The model under review builds one solid part; all positions refer to its coordinate system, in mm. A direction names the side the tool comes from. Round coordinates to 2 decimals unless told otherwise and drop trailing zeros. Order: outer loops, then holes, each group sorted by start corner. A loop starts at its lowest first (then second) coordinate and runs counter-clockwise, first axis right, second up.
```python
from build123d import *

# Parameters (mm, degrees)
SKETCH1_W                                           = 80
SKETCH1_H                                           = 100
BOSS_EXTRUDE1_DEPTH                                 = 10
SKETCH2_R                                           = 18
CUT_EXTRUDE1_DEPTH                                  = 129.452325787
SKETCH3_W                                           = 80
SKETCH3_H                                           = 46
CUT_EXTRUDE2_DEPTH                                  = 4
CBORE_FOR_M3_HEX_SOCKET_HEAD_CAP_SCREW1_D           = 3.4
CBORE_FOR_M3_HEX_SOCKET_HEAD_CAP_SCREW1_CBORE_D     = 6.5
CBORE_FOR_M3_HEX_SOCKET_HEAD_CAP_SCREW1_CBORE_DEPTH = 3.4


with BuildPart() as part:
    # Sketch1 → Boss-Extrude1 (new body)
    with BuildSketch(Plane.XY):
        with Locations((40, 50)):
            Rectangle(SKETCH1_W, SKETCH1_H)
    extrude(amount=BOSS_EXTRUDE1_DEPTH)

    # Sketch2 → Cut-Extrude1 (cut, through all)
    with BuildSketch(Plane.XY.offset(10)):
        with Locations((40, 73)):
            Circle(SKETCH2_R)
    extrude(amount=-CUT_EXTRUDE1_DEPTH, mode=Mode.SUBTRACT)

    # Sketch3 → Cut-Extrude2 (cut)
    with BuildSketch(Plane.XY.offset(10)):
        with Locations((40, 23)):
            Rectangle(SKETCH3_W, SKETCH3_H)
    extrude(amount=-CUT_EXTRUDE2_DEPTH, mode=Mode.SUBTRACT)

    # CBORE for M3 Hex Socket Head Cap Screw1 (through all)
    with Locations(Plane.XY.offset(6)):
        with Locations((8, 8), (40, 8), (72, 8), (40, 24), (72, 24), (8, 24)):
            CounterBoreHole(CBORE_FOR_M3_HEX_SOCKET_HEAD_CAP_SCREW1_D / 2, CBORE_FOR_M3_HEX_SOCKET_HEAD_CAP_SCREW1_CBORE_D / 2, CBORE_FOR_M3_HEX_SOCKET_HEAD_CAP_SCREW1_CBORE_DEPTH)


solid = part.part
```
(1) To check wall thickness, follow probe 1 along Y at (x, z) = (40, 3.35); probe 2 along Y at (x, z) = (72, 4.5); probe 3 along Y at (x, z) = (40, 2.5). State the ranges of each line that lie inside material, in increasing order.
Data:
probe 1: y = 0 to 4.75, 11.25 to 20.75, 27.25 to 55, 91 to 100
probe 2: y = 0 to 4.75, 11.25 to 20.75, 27.25 to 100
probe 3: y = 0 to 6.3, 9.7 to 22.3, 25.7 to 55, 91 to 100
(2) Consider section D-D (x = 8). Write out the cut boundary in (y, z), and give its area (3 significant figures).
Data:
outline: (0, 0) - (6.3, 0) - (6.3, 2.6) - (4.75, 2.6) - (4.75, 6) - (0, 6) - close; (9.7, 0) - (22.3, 0) - (22.3, 2.6) - (20.75, 2.6) - (20.75, 6) - (11.25, 6) - (11.25, 2.6) - (9.7, 2.6) - close; (25.7, 0) - (100, 0) - (100, 10) - (46, 10) - (46, 6) - (27.25, 6) - (27.25, 2.6) - (25.7, 2.6) - close
area: 754 mm2
(3) Insertion check: pin 1 (7 mm diameter, centred on x = 40, y = 23, fed in from +Z); pin 2 (2.5 mm diameter, centred on x = 8, y = 8, fed in from +Z); pin 3 (5 mm diameter, centred on x = 40, y = 8, fed in from +Z). Each pin has a flat end and moves straight along its axis. Give the tip position at first contact, or say it passes through.
Data:
pin 1: stops at z = 6
pin 2: passes through
pin 3: stops at z = 2.6
(4) Consider section C-C (z = 8.25). Write out the cut boundary in (x, y).
Data:
outline: (0, 46) - (80, 46) - (80, 100) - (0, 100) - close; hole circle Ø36 at (40, 73)
(5) Draft analysis for pull direction X (two halves, no side actions). For faces 1 (the cylindrical face through (43.1, 8.98, 4.32)), 2 (the flat face through (39, 28, 6)), 3 (the flat face through (0, 60, 4)), state which applies: pulls with the +X half, pulls with the -X half, needs draft (parallel to the pull), parting line crosses it, or undercut.
Data:
face 1: undercut
face 2: needs draft
face 3: pulls with the -X half
(6) Consider section A-A (y = 73). Write out the cut boundary in (x, z).
Data:
outline: (0, 0) - (22, 0) - (22, 10) - (0, 10) - close; (58, 0) - (80, 0) - (80, 10) - (58, 10) - close
(7) For faces 4 (the cylindrical face through (68.753, 8.143, 4.324)), 5 (the cylindrical face through (41.35, 6.97, 1.28)), 6 (the flat face through (39, 46, 8)), list the 3-axis set-ups (+Z, -Z, +X, -X, +Y, -Y) from which the entire face can be reached by the end or side of a thin tool; tool diameter is ignored.
Data:
face 4: +Z
face 5: +Z, -Z
face 6: +Z, +X, -X, -Y
(8) Consider section B-B (x = 40). Write out the cut boundary in (y, z).
Data:
outline: (0, 0) - (6.3, 0) - (6.3, 2.6) - (4.75, 2.6) - (4.75, 6) - (0, 6) - close; (9.7, 0) - (22.3, 0) - (22.3, 2.6) - (20.75, 2.6) - (20.75, 6) - (11.25, 6) - (11.25, 2.6) - (9.7, 2.6) - close; (25.7, 0) - (55, 0) - (55, 10) - (46, 10) - (46, 6) - (27.25, 6) - (27.25, 2.6) - (25.7, 2.6) - close; (91, 0) - (100, 0) - (100, 10) - (91, 10) - close
